For this review, take the finished solid that the model builds, in its own axes (mm). A direction names the side the tool comes from. Give positions to 0.01 mm unless a question says otherwise; leave off trailing zeros. Write each loop counter-clockwise with the first axis right and the second up, starting at its lowest first coordinate (ties: lowest second). Pieces come first, ordered by that corner, then holes. Notation, with made-up numbers: M 36.25,9 L 93.25,9 A27 ccw 93.25,43 Z; hole C 2,48 d10. An arc over 180 degrees is marked long. Write item = value, one per line.
Autodesk Inventor part; units mm, degrees
ref_plane "YZ Plane" through (0, 0, 0) normal (1, 0, 0) x (0, 1, 0)
ref_plane "XZ Plane" through (0, 0, 0) normal (0, 1, 0) x (-1, 0, 0)
ref_plane "XY Plane" through (0, 0, 0) normal (0, 0, 1) x (1, 0, 0)
sketch "Szkic1" plane through (0, 0, 0) normal (0, 1, 0) x (-1, 0, 0)
  line L0 (26.7, -27.1) -> (-26.7, -27.1)
  line L1 (-26.7, -27.1) -> (-26.7, 27.1)
  line L2 (-26.7, 27.1) -> (26.7, 27.1)
  line L3 (26.7, 27.1) -> (26.7, -27.1)
  line L4 (26.7, -27.1) -> (-26.7, 27.1) construction
  line L5 (-26.7, -27.1) -> (26.7, 27.1) construction
  point P0 (0, 0)
  dimension "d0" = 53.4
  dimension "d1" = 54.2
extrude "Wyciągnięcie proste1" add sketch "Szkic1" along normal blind 2
sketch "Szkic11" plane through (0, 2, 0) normal (0, 1, 0) x (1, 0, 0)
  line L0 (-26.7, -27.1) -> (26.7, -27.1)
  line L1 (26.7, -27.1) -> (25.9, -27.1)
  line L2 (25.9, -27.1) -> (19.5, -27.1)
  line L3 (19.5, -27.1) -> (19.5, -28.7)
  line L4 (19.5, -28.7) -> (25.9, -28.7)
  line L5 (25.9, -28.7) -> (25.9, -27.1)
  arc A0 (19.5, -28.7) -> (25.9, -28.7) centre (22.7, -28.7) ccw
  point P0 (0, 0)
  dimension "d37" = 0.8
  dimension "d38" = 6.4
  dimension "d39" = 1.6
  dimension "d40" = 3.2
extrude "Wyciągnięcie proste10" add sketch "Szkic11" against normal blind 2
sketch "Szkic12" plane through (0, 2, 0) normal (0, 1, 0) x (1, 0, 0)
  arc A0 (19.5, -28.7) -> (25.9, -28.7) centre (22.7, -28.7) ccw
  circle A1 centre (22.7, -28.7) radius 1.6
  point P0 (0, 0)
  dimension "d43" = 3.2
extrude "Wyciągnięcie proste11" cut sketch "Szkic12" against normal through all
sketch "Szkic49" plane through (0, 0, 0) normal (0, -1, 0) x (1, 0, 0)
  circle A0 centre (22.7, 28.7) radius 1.6
  circle A1 centre (22.7, 28.7) radius 1.6
  point P0 (0, 0)
extrude "Wyciągnięcie proste41" add sketch "Szkic49" against normal blind 1
sketch "Szkic50" plane through (0, 0, 0) normal (0, -1, 0) x (1, 0, 0)
  circle A0 centre (22.7, 28.7) radius 1.6
  circle A1 centre (22.7, 28.7) radius 1
  point P0 (0, 0)
  dimension "d208" = 2
extrude "Wyciągnięcie proste42" cut sketch "Szkic50" against normal blind 10 contours A1
sketch "Szkic51" plane through (0, 0, 0) normal (0, -1, 0) x (1, 0, 0)
  line L0 (5, -5) -> (-5, -5)
  line L1 (-5, -5) -> (-5, 5)
  line L2 (-5, 5) -> (5, 5)
  line L3 (5, 5) -> (5, -5)
  line L4 (5, -5) -> (-5, 5) construction
  line L5 (-5, -5) -> (5, 5) construction
  point P0 (0, 0)
  dimension "d211" = 10
  dimension "d212" = 10
extrude "Wyciągnięcie proste43" add sketch "Szkic51" along normal blind 1.6
sketch "Szkic52" plane through (0, 2, 0) normal (0, 1, 0) x (1, 0, 0)
  line L0 (-25.9, 26.3) -> (-21.9, 26.3)
  line L1 (-21.9, 26.3) -> (-21.9, 22.3)
  line L2 (-21.9, 22.3) -> (-25.9, 22.3)
  line L3 (-25.9, 22.3) -> (-25.9, 26.3)
  line L4 (21.9, 26.3) -> (25.9, 26.3)
  line L5 (25.9, 26.3) -> (25.9, 22.3)
  line L6 (25.9, 22.3) -> (21.9, 22.3)
  line L7 (21.9, 22.3) -> (21.9, 26.3)
  line L8 (-25.9, -21.5) -> (-21.9, -21.5)
  line L9 (-21.9, -21.5) -> (-21.9, -25.5)
  line L10 (-21.9, -25.5) -> (-25.9, -25.5)
  line L11 (-25.9, -25.5) -> (-25.9, -21.5)
  line L12 (21.9, -21.5) -> (25.9, -21.5)
  line L13 (25.9, -21.5) -> (25.9, -25.5)
  line L14 (25.9, -25.5) -> (21.9, -25.5)
  line L15 (21.9, -25.5) -> (21.9, -21.5)
  line L16 (-25.9, 26.3) -> (-26.7, 26.3)
  line L17 (-25.9, -21.5) -> (-26.7, -21.5)
  line L18 (25.9, 26.3) -> (26.7, 26.3)
  line L19 (25.9, -21.5) -> (26.7, -21.5)
  line L20 (26.7, -27.1) -> (26.7, 27.1)
  line L21 (-26.7, 27.1) -> (-26.7, -27.1)
  line L22 (-25.9, 26.3) -> (-25.9, 27.1)
  line L23 (25.9, 26.3) -> (25.9, 27.1)
  line L24 (26.7, -27.1) -> (26.7, 27.1)
  line L25 (25.9, 26.3) -> (26.7, 26.3) construction
  line L26 (26.7, 27.1) -> (-26.7, 27.1)
  line L27 (-25.9, -25.5) -> (-25.9, -27.1)
  line L28 (-26.7, 27.1) -> (-26.7, -27.1)
  line L29 (-25.9, -25.5) -> (-24.3, -25.5) construction
  line L30 (25.9, -25.5) -> (25.9, -27.1)
  line L31 (-26.7, -27.1) -> (19.5, -27.1)
  point P0 (0, 0)
  dimension "d215" = 4
  dimension "d216" = 4
  dimension "d217" = 4
  dimension "d218" = 4
  dimension "d219" = 4
  dimension "d220" = 4
  dimension "d221" = 4
  dimension "d222" = 4
  dimension "d223" = 0.8
  dimension "d224" = 0.8
  dimension "d225" = 0.8
  dimension "d226" = 0.8
  dimension "d227" = 0.8
  dimension "d228" = 0.8
  dimension "d229" = 90
  dimension "d230" = 1.6
  dimension "d231" = 90
  dimension "d232" = 1.6
extrude "Wyciągnięcie proste44" cut sketch "Szkic52" against normal up to surface (2 mm away) contours L0 L1 L2 L3 | L13 L14 L15 L12 | L5 L6 L7 L4 | L8 L9 L10 L11
properties part number "PMS3003_dol"
1. The part is to be moulded in two halves that separate along X. For faces 6 (the face through (-24, 1, -26.3)), 7 (the face through (-3, 1, 27.1)), 8 (the face through (25.9, 1, 28)), 9 (the face through (-5, -1, 0)), say which applies: +X half, -X half, draft (parallel to the pull), parting line (faces both ways), or undercut.
Responses:
face_6 = undercut
face_7 = draft
face_8 = +X half
face_9 = -X half
2. We need section C-C, the plane z = -9. Write out the cut boundary in (x, y).
Responses:
outline = M -26.7,0 L 26.7,0 L 26.7,2 L -26.7,2 Z
3. Machinability: for faces 1 (the face through (0, -1, -5)), 2 (the face through (0, -1.6, 0)), 3 (the face through (-21.9, 1, 23)), 4 (the face through (22.6, 1, 31.9)), 5 (the face through (5, -1, 0)), which of the approach directions +Z, -Z, +X, -X, +Y, -Y give a long, thin tool a straight path to every point of the face, cutting with its end or side? Answer none if there is none.
Responses:
face_1 = -Z, +X, -X, -Y
face_2 = +Z, -Z, +X, -X, -Y
face_3 = +Y, -Y
face_4 = +Z, +Y, -Y
face_5 = +Z, -Z, +X, -Y
4. We need section A-A, the plane x = 22.7. Write out the cut boundary in (y, z), then the cut area to 3 significant figures.
Responses:
outline = M 0,-27.1 L 2,-27.1 L 2,-26.3 L 0,-26.3 Z; M 0,-22.3 L 2,-22.3 L 2,21.5 L 0,21.5 Z; M 0,25.5 L 2,25.5 L 2,27.1 L 1,27.1 L 1,27.7 L 0,27.7 Z; M 0,29.7 L 1,29.7 L 1,30.3 L 2,30.3 L 2,31.9 L 0,31.9 Z
area = 96.8 mm2
5. We need section B-B, the plane x = 1. Write out the cut boundary in (y, z).
Responses:
outline = M -1.6,-5 L 0,-5 L 0,-27.1 L 2,-27.1 L 2,27.1 L 0,27.1 L 0,5 L -1.6,5 Z
6. We need section D-D, the plane y = -0.95. Write out the cut boundary in (x, z), then the cut area to 3 significant figures.
Responses:
outline = M -5,-5 L 5,-5 L 5,5 L -5,5 Z
area = 100 mm2
7. For line 1 along Z through (x, y) = (22.7, 1.65); line 2 along X through (y, z) = (1.25, 23); line 3 along Z through (x, y) = (22.7, 0.6), list the stretches that pass through material, from the lowest coordinate up. Write a range as from..to.
Responses:
line_1 = -27.1..-26.3, -22.3..21.5, 25.5..27.1, 30.3..31.9
line_2 = -26.7..-25.9, -21.9..21.9, 25.9..26.7
line_3 = -27.1..-26.3, -22.3..21.5, 25.5..27.7, 29.7..31.9
8. Insertion check: P1, Ø1.3, axis at y = -0.5, z = 1, coming from the -X side; P2, Ø1.6, axis at x = 24.5, y = 1, coming from the +Z side; P3, Ø1.6, axis at x = -23, y = 1, coming from the +Z side; P4, Ø0.5, axis at x = 1, y = -1, coming from the -Z side. Each pin has a flat end and moves straight along its axis. Give the tip position at first contact, or say it passes through.
Responses:
P1 = -26.7
P2 = 31.74
P3 = 27.1
P4 = -5
